```python
from build123d import *

# Parameters (mm, degrees)
BOSS_EXTRUDE1_DEPTH = 40
SKETCH2_W           = 9.5
SKETCH2_H           = 1.5
SKETCH2_W_2         = 5
CUT_EXTRUDE1_DEPTH  = 6
SKETCH2_3_W         = 9.5
SKETCH2_3_H         = 9.25
SKETCH2_3_W_2       = 5
BOSS_EXTRUDE2_DEPTH = 13
BOSS_EXTRUDE3_DEPTH = 3


with BuildPart() as part:
    # Sketch1 → Boss-Extrude1 (new body, symmetric)
    with BuildSketch(Plane(origin=(0, 0, 0), x_dir=(1, 0, 0), z_dir=(0, 1, 0))):
        with BuildLine():
            Line((-7.25, 3), (-2.25, 3))
            Line((-2.25, 3), (-2.25, 0))
            ThreePointArc((-2.25, 0), (0, -2.25), (2.25, 0))
            Line((2.25, 0), (2.25, 3))
            Line((2.25, 3), (7.25, 3))
            Line((7.25, 3), (7.25, -10))
            Line((7.25, -10), (-7.25, -10))
            Line((-7.25, -10), (-7.25, 3))
        make_face()
    extrude(amount=BOSS_EXTRUDE1_DEPTH, both=True)

    # Sketch2 → Cut-Extrude1 (cut)
    with BuildSketch(Plane(origin=(0, 0, -3), x_dir=(-1, 0, 0), z_dir=(0, 0, -1))):
        with Locations((2.5, 30)):
            Rectangle(SKETCH2_W, SKETCH2_H)
        with Locations((-4.75, 30)):
            Rectangle(SKETCH2_W_2, SKETCH2_H)
    extrude(amount=-CUT_EXTRUDE1_DEPTH, mode=Mode.SUBTRACT)

    # Sketch2_3 → Boss-Extrude2 (add, through all)
    with BuildSketch(Plane(origin=(0, 0, -3), x_dir=(-1, 0, 0), z_dir=(0, 0, -1))):
        with Locations((2.5, -35.375)):
            Rectangle(SKETCH2_3_W, SKETCH2_3_H)
        with Locations((-4.75, -35.375)):
            Rectangle(SKETCH2_3_W_2, SKETCH2_3_H)
    extrude(amount=-BOSS_EXTRUDE2_DEPTH)

    # Sketch3 → Boss-Extrude3 (add)
    with BuildSketch(Plane(origin=(0, -30.75, 0), x_dir=(1, 0, 0), z_dir=(0, 1, 0))):
        with BuildLine():
            Line((2.25, 0), (2.25, 3))
            Line((2.25, 3), (-2.25, 3))
            Line((-2.25, 3), (-2.25, 0))
            ThreePointArc((-2.25, 0), (0, 2.25), (2.25, 0))
        make_face()
    extrude(amount=BOSS_EXTRUDE3_DEPTH)


solid = part.part
```
Source: CAD feature listing. Evaluate the final solid. Frame: model axes, mm. A direction names the side the tool comes from. Round coordinates to 2 decimals unless told otherwise and drop trailing zeros. Loops run counter-clockwise (first coordinate to the right, second up) from the corner with the lowest first, then second, coordinate; pieces in that order, holes last. Notation, with made-up numbers: (-16.75, -6) - (4.25, -6) arc R21 ccw to (4.25, 31) - close; hole circle Ø7 at (-1.75, -8.5). An arc over 180 degrees is marked (long way). Use CSV: the item, a comma, the result in double quotes.
Q1. Section query C-C, the plane y = -6.5. Output: boundary loops of the cut face in (x, z), then the cut area to 3 significant figures.
Reported:
outline,"(-7.25, -3) - (-2.25, -3) - (-2.25, 0) arc R2.25 cw to (2.25, 0) - (2.25, -3) - (7.25, -3) - (7.25, 10) - (-7.25, 10) - close"
area,"167 mm^2"
Q2. Section query B-B, the plane x = 0. Output: boundary loops of the cut face in (y, z).
Reported:
outline,"(-40, -3) - (-27.75, -3) - (-27.75, -2.25) - (-30.75, -2.25) - (-30.75, 2.25) - (29.25, 2.25) - (29.25, 3) - (30.75, 3) - (30.75, 2.25) - (40, 2.25) - (40, 10) - (-40, 10) - close"
Q3. Reachability of faces 1 (the flat face through (-2.25, 1, -2)), 2 (the cylindrical face through (-1.038, -1.17, 1.996)), 3 (the flat face through (0, 1, 10)), 4 (the flat face through (2, 30.75, 2)) from +Z, -Z, +X, -X, +Y, -Y: full face, straight path, thin tool, end or side. Return the list, or none.
Reported:
face 1,"-Z, +Y"
face 2,"+Y"
face 3,"+Z, +X, -X, +Y, -Y"
face 4,"-Z, +X, -X"
Q4. Section query A-A, the plane z = 0.75. Output: boundary loops of the cut face in (x, y).
Reported:
outline,"(-7.25, -40) - (7.25, -40) - (7.25, 29.25) - (2.12, 29.25) - (2.12, -30.75) - (-2.12, -30.75) - (-2.12, 29.25) - (-7.25, 29.25) - close; (-7.25, 30.75) - (-2.12, 30.75) - (-2.12, 40) - (-7.25, 40) - close; (2.12, 30.75) - (7.25, 30.75) - (7.25, 40) - (2.12, 40) - close"
Q5. Mould query, pull axis X, two halves, no side actions, for faces 5 (the flat face through (7.25, 1, 3)), 6 (the flat face through (0, -40, 3)), 7 (the flat face through (2.25, 35, -1)). Classes: pulls with the +X half, pulls with the -X half, needs draft (parallel to the pull), parting line crosses it, or undercut.
Reported:
face 5,"pulls with the +X half"
face 6,"needs draft"
face 7,"undercut"
Q6. Pin query (flat end, axial travel): pin 1 Ø1.3 at (x, z) = (-0.5, 0) entering from +Y; pin 2 Ø6.5 at (x, z) = (-2, -0.5) entering from +Y; pin 3 Ø0.8 at (x, y) = (0.5, 30) entering from -Z. Return the tip coordinate at first contact, or that it passes through.
Reported:
pin 1,"y = -30.75"
pin 2,"y = 40"
pin 3,"z = 3"
Q7. Ray query, line 1 along X through (y, z) = (10.5, 0); line 2 along Y through (x, z) = (-4.75, -0.5); line 3 along X through (y, z) = (-25, 0.75). Return the intervals inside material, ascending.
Reported:
line 1,"-7.25 to -2.25, 2.25 to 7.25"
line 2,"-40 to 29.25, 30.75 to 40"
line 3,"-7.25 to -2.12, 2.12 to 7.25"
